```python
from build123d import *

# Parameters (mm, degrees)
F0_R     = 1.45
F1_DEPTH = 5
F2_R     = 1.75
F3_DEPTH = 25
F4_W     = 8
F4_H     = 6
F4_R     = 1.45
F5_DEPTH = 3
F6_R     = 3.5
F7_DEPTH = 2


with BuildPart() as f1:
    # F0 (on Top) → F1 (new body)
    with BuildSketch(Plane.XY):
        Polygon((0, 30), (0, 0), (20, 0), (20, 60), (0, 60), (0, 46), (-18, 46), (-18, 30), align=None)
        with Locations((-14.043072, 33.05522)):
            Circle(F0_R, mode=Mode.SUBTRACT)
        with Locations((4.956928, 33.05522)):
            Circle(F0_R, mode=Mode.SUBTRACT)
    extrude(amount=F1_DEPTH)

    # F2 (on face) → F3 (cut)
    with BuildSketch(Plane.XY.offset(5)):
        with Locations((10.002809, 51.71774)):
            Circle(F2_R)
        with Locations((10.166974, 5.901501)):
            Circle(F2_R)
    extrude(amount=-F3_DEPTH, mode=Mode.SUBTRACT)

    # F4 (on face) → F5 (join)
    with BuildSketch(Plane.XY.offset(5)):
        with Locations((-14, 33)):
            Rectangle(F4_W, F4_H)
        with Locations((-14.043072, 33.05522)):
            Circle(F4_R, mode=Mode.SUBTRACT)
        with Locations((6.67554, 33)):
            Rectangle(F4_W, F4_H)
        with Locations((4.956928, 33.05522)):
            Circle(F4_R, mode=Mode.SUBTRACT)
    extrude(amount=F5_DEPTH)

    # F6 (on face) → F7 (cut)
    with BuildSketch(Plane.XY.offset(5)):
        with Locations((10.002809, 51.71774)):
            Circle(F6_R)
        with Locations((10.166974, 5.901501)):
            Circle(F6_R)
    extrude(amount=-F7_DEPTH, mode=Mode.SUBTRACT)


solid = f1.part
```
Input: part model. Units: mm. Frame: model coordinates. A direction names the side the tool comes from. Coordinates: 2 decimals unless noted, no trailing zeros. Write each loop counter-clockwise with the first axis right and the second up, starting at its lowest first coordinate (ties: lowest second). Pieces come first, ordered by that corner, then holes.
1) Section C-C on x = -11.5. Output: boundary loops of the cut face in (y, z).
2) Material intervals for line 1 along X through (y, z) = (52, 3.75); line 2 along X through (y, z) = (33.5, 6); line 3 along Z through (x, y) = (9, 22.5), sorted ascending.
3) Mould query, pull axis X, two halves, no side actions, for faces 1 (the flat face through (20, 30, 2)), 2 (the cylindrical face through (-14.36, 31.64, 3.94)), 3 (the cylindrical face through (13.505, 6.953, 4.014)), 4 (the flat face through (-9, 30, 3)). Classes: pulls with the +X half, pulls with the -X half, needs draft (parallel to the pull), parting line crosses it, or undercut.
4) Pin query (flat end, axial travel): pin 1 Ø2.5 at (y, z) = (12, 2.5) entering from -X; pin 2 Ø12 at (x, y) = (15, 22.5) entering from +Z; pin 3 Ø5.5 at (x, y) = (10.5, 51.5) entering from +Z. Return the tip coordinate at first contact, or that it passes through.
5) Section A-A on z = 6. Output: boundary loops of the cut face in (x, y).
6) Set-up query: faces 5 (the flat face through (10.676, 33, 6)), 6 (the flat face through (-14, 36, 6)), 7 (the flat face through (-9, 46, 2)), 8 (the cylindrical face through (4.64, 31.64, 3.94)), 9 (the flat face through (8, 51, 3)). Return all of +Z, -Z, +X, -X, +Y, -Y with unobstructed straight access to the full face (end or side cutting, diameter ignored); none if empty.
7) Section B-B on y = 7. Output: boundary loops of the cut face in (x, z), and give its area (3 significant figures).
8) Section D-D on x = 5. Output: boundary loops of the cut face in (y, z), and give its area (3 significant figures).
Check result:
1. outline: (30, 0) - (46, 0) - (46, 5) - (36, 5) - (36, 8) - (30, 8) - close
2. line 1: x = 0 to 6.51, 13.49 to 20
2. line 2: x = -18 to -15.42, -12.66 to -10, 2.68 to 3.58, 6.34 to 10.68
2. line 3: z = 0 to 5
3. face 1: pulls with the +X half
3. face 2: undercut
3. face 3: undercut
3. face 4: needs draft
4. pin 1: stops at x = 0
4. pin 2: stops at z = 5
4. pin 3: stops at z = 3
5. outline: (-18, 30) - (-10, 30) - (-10, 36) - (-18, 36) - close; (2.68, 30) - (10.68, 30) - (10.68, 36) - (2.68, 36) - close; hole circle Ø2.9 at (-14.04, 33.06); hole circle Ø2.9 at (4.96, 33.06)
6. face 5: +Z, +X, +Y, -Y
6. face 6: +Z, +X, -X, +Y
6. face 7: +Z, -Z, -X, +Y
6. face 8: +Z, -Z
6. face 9: +Z
7. outline: (0, 0) - (8.8, 0) - (8.8, 3) - (6.84, 3) - (6.84, 5) - (0, 5) - close; (11.53, 0) - (20, 0) - (20, 5) - (13.49, 5) - (13.49, 3) - (11.53, 3) - close
7. area: 78.5 mm2
8. outline: (0, 0) - (31.61, 0) - (31.61, 8) - (30, 8) - (30, 5) - (0, 5) - close; (34.5, 0) - (60, 0) - (60, 5) - (36, 5) - (36, 8) - (34.5, 8) - close
8. area: 295 mm2
